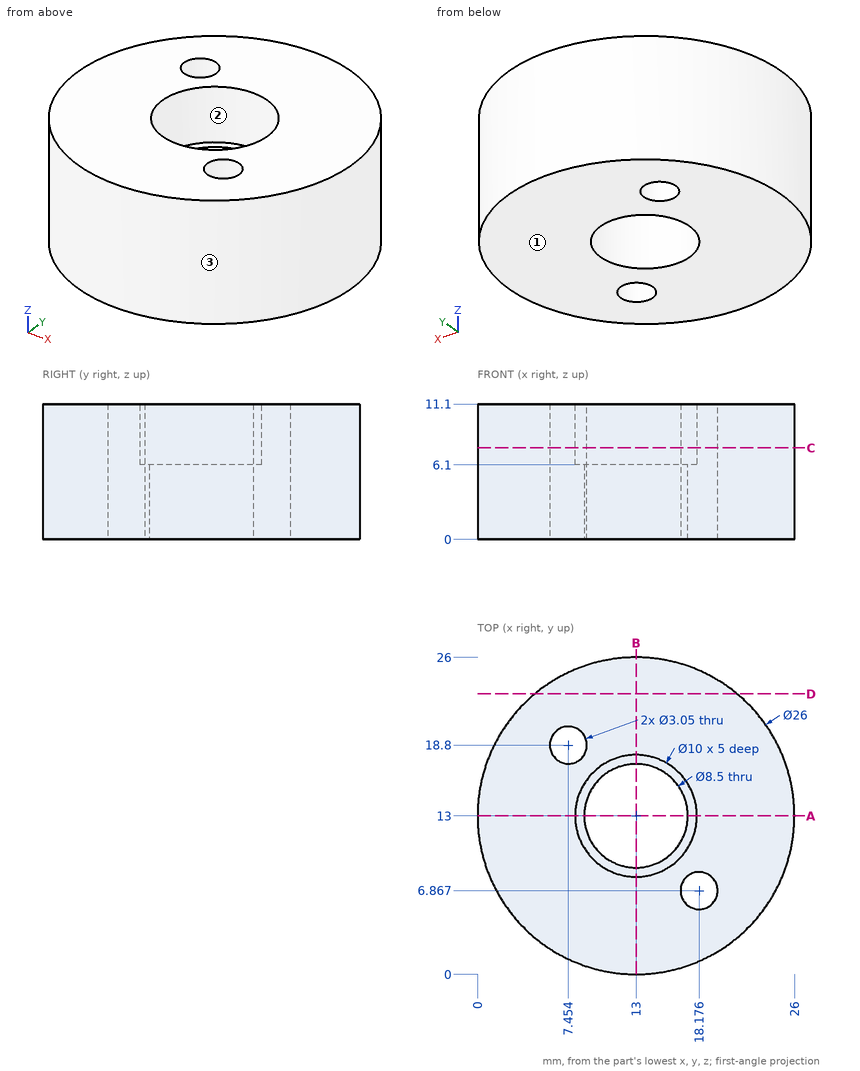
Job drawing, mm, ordinate dimensions from the low corner. One solid piece. Give positions to 0.01 mm unless a question says otherwise; leave off trailing zeros. Loops run counter-clockwise (first coordinate to the right, second up) from the corner with the lowest first, then second, coordinate; pieces in that order, holes last. Notation, with made-up numbers: M 80.25,84.25 L 98.25,84.25 A14 ccw 98.25,102.25 Z; hole C -17.75,-10.5 d8. An arc over 180 degrees is marked long. Answer in a Markdown table with one row per item. Add a question column.
Item 1: Band-saw the part on C-C on z = 7.5. Give the number of separate pieces and of enclosed holes in the cut face, then the cut area to 3 significant figures.
Item 2: Probe probe 1 along Y at (x, z) = (14, 4.5); probe 2 along Y at (x, z) = (10, 0.75); probe 3 along X at (y, z) = (16.5, 2). List the from-to ranges inside material, lowest first.
Item 3: Mould opens along X. For the marked faces 1, 2 and 3 say: +X half, -X half, draft (parallel to the pull), parting line (faces both ways), or undercut.
Item 4: Band-saw the part on A-A on y = 13. Give the cut face in (x, z), then the cut area to 3 significant figures.
Item 5: Drop flat-ended pins along their axis: P1, Ø5, axis at x = 7.45, y = 18.8, coming from the +Z side; P2, Ø6, axis at x = 13, y = 13, coming from the -Z side; P3, Ø6, axis at x = 9.5, z = 9.5, coming from the +Y side; P4, Ø6, axis at x = 22, z = 5, coming from the -Y side. Give the stop position or say it passes through.
Item 6: Band-saw the part on D-D on y = 23. Give the cut face in (x, z), then the cut area to 3 significant figures.
Reply:
| question | item | result |
|---|---|---|
| 1 | separate pieces | 1 |
| 1 | enclosed holes | 3 |
| 1 | area | 438 mm^2 |
| 2 | probe 1 | y = 0.04 to 8.87, 17.13 to 25.96 |
| 2 | probe 2 | y = 0.35 to 9.99, 16.01 to 25.65 |
| 2 | probe 3 | x = 0.48 to 10.59, 15.41 to 25.52 |
| 3 | face 1 | draft |
| 3 | face 2 | undercut |
| 3 | face 3 | parting line |
| 4 | outline | M 0,0 L 8.75,0 L 8.75,6.1 L 8,6.1 L 8,11.1 L 0,11.1 Z; M 17.25,0 L 26,0 L 26,11.1 L 18,11.1 L 18,6.1 L 17.25,6.1 Z |
| 4 | area | 187 mm^2 |
| 5 | P1 | stops at z = 11.1 |
| 5 | P2 | passes through |
| 5 | P3 | stops at y = 25.99 |
| 5 | P4 | stops at y = 1.47 |
| 6 | outline | M 4.69,0 L 21.31,0 L 21.31,11.1 L 4.69,11.1 Z |
| 6 | area | 184 mm^2 |
